from build123d import *

# Parameters (mm, degrees)
SKETCH_1_W          = 15
SKETCH_1_H          = 15
SKETCH_1_W_2        = 13
SKETCH_1_H_2        = 13
EXTRUDE_1_DEPTH     = 112
SKETCH_3_R          = 2.2
CUT_EXTRUDE_1_DEPTH = 55


with BuildPart() as part:
    # 草图1 → 凸台-拉伸1 (new body)
    with BuildSketch(Plane.XY):
        Rectangle(SKETCH_1_W, SKETCH_1_H)
        Rectangle(SKETCH_1_W_2, SKETCH_1_H_2, mode=Mode.SUBTRACT)
    extrude(amount=EXTRUDE_1_DEPTH)

    # 草图3 → 切除-拉伸1 (cut)
    with BuildSketch(Plane(origin=(7.5, 0, 0), x_dir=(0, 0, -1), z_dir=(1, 0, 0))):
        with Locations((-15, 0)):
            Circle(SKETCH_3_R)
        with Locations((-30, 0)):
            Circle(SKETCH_3_R)
        with Locations((-97, 0)):
            Circle(SKETCH_3_R)
        with Locations((-82, 0)):
            Circle(SKETCH_3_R)
    extrude(amount=-CUT_EXTRUDE_1_DEPTH, mode=Mode.SUBTRACT)


solid = part.part
Input: part model. Units: mm. Frame: model coordinates. A direction names the side the tool comes from. Round coordinates to 2 decimals unless told otherwise and drop trailing zeros. Order: outer loops, then holes, each group sorted by start corner. A loop starts at its lowest first (then second) coordinate and runs counter-clockwise, first axis right, second up.
1. Cut plane B-B, the plane z = 97. Output: boundary loops of the cut face in (x, y).
The answers:
outline: (-7.5, -7.5) - (7.5, -7.5) - (7.5, -2.2) - (6.5, -2.2) - (6.5, -6.5) - (-6.5, -6.5) - (-6.5, -2.2) - (-7.5, -2.2) - close; (-7.5, 2.2) - (-6.5, 2.2) - (-6.5, 6.5) - (6.5, 6.5) - (6.5, 2.2) - (7.5, 2.2) - (7.5, 7.5) - (-7.5, 7.5) - close
2. Cut plane D-D, the plane y = 0. State how many separate pieces and enclosed holes the cut face has, then the cut area to 3 significant figures.
The answers:
separate pieces: 10
enclosed holes: 0
area: 189 mm2
3. Material intervals for line 1 (Y direction, x = -6.95, z = 30); line 2 (Y direction, x = 0, z = 72), sorted ascending.
The answers:
line 1: y = -7.5 to -2.2, 2.2 to 7.5
line 2: y = -7.5 to -6.5, 6.5 to 7.5
4. Mould query, pull axis Y, two halves, no side actions, for faces 3 (the face through (0, -7.5, 55)), 4 (the face through (-6.993, 0.097, 32.198)), 5 (the face through (-7, 0, 112)). Classes: released by +Y, released by -Y, zero draft, split by the parting line, or undercut.
The answers:
face 3: released by -Y
face 4: undercut
face 5: zero draft
5. Set-up query: faces 1 (the face through (6.5, 0, 55)), 2 (the face through (7.007, -0.843, 12.968)). Return all of +Z, -Z, +X, -X, +Y, -Y with unobstructed straight access to the full face (end or side cutting, diameter ignored); none if empty.
The answers:
face 1: +Z, -Z
face 2: +X, -X
6. Cut plane A-A, the plane x = -4.75. Output: boundary loops of the cut face in (y, z), then the cut area to 3 significant figures.
The answers:
outline: (-7.5, 0) - (-6.5, 0) - (-6.5, 112) - (-7.5, 112) - close; (6.5, 0) - (7.5, 0) - (7.5, 112) - (6.5, 112) - close
area: 224 mm2
